Verification items for the finished model (mm, model axes). A direction names the side the tool comes from. Coordinates: 2 decimals unless noted, no trailing zeros. Loops run counter-clockwise (first coordinate to the right, second up) from the corner with the lowest first, then second, coordinate; pieces in that order, holes last. Notation, with made-up numbers: (6.25, -32) -> (62.25, -32) arc R35 ccw to (62.25, 4) -> close; hole circle Ø9 at (51.5, -13). An arc over 180 degrees is marked (long way). Write item = value, one per line.
```python
from build123d import *

# Parameters (mm, degrees)
F0_W     = 6.35
F0_H     = 127
F1_DEPTH = 11.50874
F2_W     = 3.175
F2_H     = 3.175
F3_DEPTH = 127
F4_R     = 1.35255
F5_DEPTH = 3.175


with BuildPart() as f1:
    # F0 (on Top) → F1 (new body)
    with BuildSketch(Plane.XY):
        with Locations((-3.175, -63.5)):
            Rectangle(F0_W, F0_H)
    extrude(amount=F1_DEPTH)

    # F2 (on face) → F3 (cut, through all)
    with BuildSketch(Plane.XZ.offset(127)):
        with Locations((-1.5875, 9.92124)):
            Rectangle(F2_W, F2_H)
    extrude(amount=-F3_DEPTH, mode=Mode.SUBTRACT)

    # F4 (on face) → F5 (cut)
    with BuildSketch(Plane(origin=(0, 0, 0), x_dir=(1, 0, 0), z_dir=(0, 0, -1))):
        with Locations((-3.175, 123.825)):
            Circle(F4_R)
        with Locations((-3.175, 63.5)):
            Circle(F4_R)
        with Locations((-3.175, 3.175)):
            Circle(F4_R)
    extrude(amount=-F5_DEPTH, mode=Mode.SUBTRACT)


solid = f1.part
```
1) Tool access check on faces 1 (the face through (-2, -64, 8.334)), 2 (the face through (-1.8, -62.6, 0)), 3 (the face through (-3, -124, 3.175)). Record the directions out of +Z, -Z, +X, -X, +Y, -Y that give a thin tool (end or side, any length) a straight path to the whole face; none if there is none.
Ans:
face_1 = +Z, +X, +Y, -Y
face_2 = -Z, +X, -X, +Y, -Y
face_3 = -Z
2) Sectioned sample at C-C, the plane y = -63.5. Record the cut outline in (x, z) (3 decimals), plus the area to 3 significant figures.
Ans:
outline = (-6.35, 0) -> (-4.528, 0) -> (-4.528, 3.175) -> (-1.822, 3.175) -> (-1.822, 0) -> (0, 0) -> (0, 8.334) -> (-3.175, 8.334) -> (-3.175, 11.509) -> (-6.35, 11.509) -> close
area = 54.4 mm2
3) Release check for a two-part mould opening along X. For faces 4 (the face through (-2.55, -62.3, 1.57)), 5 (the face through (-5, -63, 11.509)), 6 (the face through (-3.175, -64, 10)) record: pulls with the +X half, pulls with the -X half, needs draft (parallel to the pull), parting line crosses it, or undercut.
Ans:
face_4 = undercut
face_5 = needs draft
face_6 = pulls with the +X half
4) Material ranges on line 1 (Z direction, x = -2.25, y = -38.5); line 2 (Y direction, x = -3.75, z = 2.75), recorded low to high.
Ans:
line_1 = 0 to 8.33
line_2 = -127 to -125.05, -122.6 to -64.72, -62.28 to -4.4, -1.95 to 0
5) Depth check by flat-ended pin: pin 1 Ø3 at (x, y) = (-5.5, -22.5) entering from -Z; pin 2 Ø0.8 at (x, y) = (-3.5, -63) entering from -Z (3 decimals); pin 3 Ø1.6 at (x, y) = (-2, -87) entering from +Z. Enter the tip coordinate at first touch or a pass-through.
Ans:
pin_1 = 0
pin_2 = 3.175
pin_3 = 8.33
6) Sectioned sample at A-A, the plane y = -28. Record the cut outline in (x, z) (3 decimals), plus the area to 3 significant figures.
Ans:
outline = (-6.35, 0) -> (0, 0) -> (0, 8.334) -> (-3.175, 8.334) -> (-3.175, 11.509) -> (-6.35, 11.509) -> close
area = 63.0 mm2
7) Sectioned sample at B-B, the plane z = 9.5. Record the cut outline in (x, y) (3 decimals), plus the area to 3 significant figures.
Ans:
outline = (-6.35, -127) -> (-3.175, -127) -> (-3.175, 0) -> (-6.35, 0) -> close
area = 403 mm2
